Autodesk Inventor part; units mm, degrees
ref_plane "Płaszczyzna konstrukcyjna1" through (0, 0, 17) normal (-1, 0, 0) x (0, 0, 1)
ref_plane "YZ Plane" through (0, 0, 0) normal (1, 0, 0) x (0, 1, 0)
ref_plane "XZ Plane" through (0, 0, 0) normal (0, 1, 0) x (-1, 0, 0)
sketch "Szkic1" plane through (0, 0, 0) normal (0, 1, 0) x (-1, 0, 0)
  line L0 (0, 17) -> (0, -17) construction
  line L1 (0, 0) -> (-17, 0)
  line L2 (0, 17) -> (0, 19)
  line L3 (0, -17) -> (0, -19)
  line L4 (-16.5569, 0) -> (-18.5569, 0)
  line L5 (0, 19) -> (0, 29)
  line L6 (0, 29) -> (-2, 29)
  line L7 (-2, 29) -> (-2, 18.7083)
  line L8 (0, -19) -> (0, -29)
  line L9 (0, -29) -> (-2, -29)
  line L10 (-2, -29) -> (-2, -18.8469)
  line L11 (-18.5573, 2.8889) -> (-18.5573, -3.1111)
  arc A0 (-2, 18.7083) -> (-18.5573, 2.8889) centre (-2.7215, 2.8889) ccw
  arc A1 (-18.5573, -3.1111) -> (-2, -18.8469) centre (-2.8011, -3.1111) ccw
  arc A2 (0, 17) -> (0, -17) centre (0.449, 0) ccw
  dimension "d0" = 34
  dimension "d1" = 17
  dimension "d2" = 2
  dimension "d3" = 2
  dimension "d4" = 2
  dimension "d5" = 10
  dimension "d6" = 2
  dimension "d7" = 10
  dimension "d8" = 2
  dimension "d41" = 6
ref_plane "Płaszczyzna konstrukcyjna1" through (0, 0, 17) normal (-1, 0, 0) x (0, 0, 1)
extrude "Wyciągnięcie proste3" add sketch "Szkic1" along normal blind 10
sketch "Szkic4" plane through (0, 0, -29) normal (-1, 0, 0) x (0, 0, 1)
  line L0 (10.1531, 0) -> (10.1531, 10)
  line L1 (10.1531, 5) -> (0, 5) construction
  line L2 (0, 0) -> (0, 10)
  line L3 (10.1531, 10) -> (0, 10)
  line L4 (5.0765, 10) -> (5.0765, 0) construction
  line L5 (10.1531, 0) -> (0, 0)
  line L6 (47.7083, 0) -> (47.7083, 10)
  line L7 (47.7083, 5) -> (58, 5) construction
  line L8 (58, 0) -> (58, 10)
  line L9 (46, 10) -> (58, 10)
  line L10 (52.8541, 10) -> (52.8541, 0) construction
  circle A0 centre (52.8541, 5) radius 3
  circle A1 centre (5.0765, 5) radius 3
  point P0 (29, 0)
  dimension "d45" = 6
  dimension "d46" = 6
hole "Otwór4" at (0, 5, -23.9235) at (0, 5, 23.8541) direction (1, 0, 0) diameter 4.9784 depth 19.05 tip angle 118
sketch "Szkic5" plane through (18.5573, 0, 2.8889) normal (1, 0, 0) x (0, 0, -1)
  line L0 (0, 10) -> (6, 10)
  line L1 (3, 10) -> (3, 0)
  line L2 (0, 0) -> (6, 0)
  line L3 (0, 0) -> (0, 10)
  line L4 (0, 5) -> (6, 5)
  line L5 (6, 0) -> (6, 10)
  circle A0 centre (3, 5) radius 3
  point P0 (2.8889, 0)
  dimension "d54" = 6
hole "Otwór5" at (18.5573, 5, -0.1111) direction (-1, 0, 0) diameter 4.9784 depth 19.05 tip angle 118
properties part number "obejma_fi32_L44"
Design review of the part built by this model. Coordinates are the model's own, in mm. A direction names the side the tool comes from. Give positions to 0.01 mm unless a question says otherwise; leave off trailing zeros. Loops run counter-clockwise (first coordinate to the right, second up) from the corner with the lowest first, then second, coordinate; pieces in that order, holes last. Notation, with made-up numbers: (16, 77.5) -> (29, 77.5) arc R23 cw to (29, 96.5) -> close; hole circle Ø4 at (76, 16). An arc over 180 degrees is marked (long way). One line per item, written item: value.
Q1. We need section A-A on x = 8.25. Give the boundary of the cut face in (y, z).
Numbers:
outline: (0, -17.9) -> (10, -17.9) -> (10, -14.61) -> (0, -14.61) -> close; (0, 14.61) -> (10, 14.61) -> (10, 17.73) -> (0, 17.73) -> close
Q2. Draft analysis for pull direction Y (two halves, no side actions). For faces 1 (the flat face through (1, 5, -29)), 2 (the flat face through (17, 10, 0)), 3 (the flat face through (17, 0, 0)), 4 (the cylindrical face through (17.44, 7.43, 0.43)), state which applies: pulls with the +Y half, pulls with the -Y half, needs draft (parallel to the pull), parting line crosses it, or undercut.
Numbers:
face 1: needs draft
face 2: pulls with the +Y half
face 3: pulls with the -Y half
face 4: undercut
Q3. For pin 1 Ø2 at (y, z) = (5.5, -5.5) entering from -X; pin 2 Ø1 at (y, z) = (3, 0.5) entering from +X; pin 3 Ø4 at (x, y) = (11, 1.5) entering from +Z; pin 4 Ø5 at (y, z) = (4.5, -24.5) entering from +X, all flat-tipped, find the tip position at first contact; note any pin that passes through.
Numbers:
pin 1: stops at x = 15.27
pin 2: stops at x = 18.56
pin 3: stops at z = 17.43
pin 4: stops at x = 2
Q4. We need section C-C on y = 5. Give the boundary of the cut face in (x, z), and give its area (3 significant figures).
Numbers:
outline: (0, -29) -> (2, -29) -> (2, -26.41) -> (0, -26.41) -> close; (0, -21.43) -> (2, -21.43) -> (2, -18.85) arc R15.76 ccw to (18.56, -3.11) -> (18.56, -2.6) -> (16.36, -2.6) arc R17.01 cw to (0, -17) -> close; (0, 17) arc R17.01 cw to (16.39, 2.38) -> (18.56, 2.38) -> (18.56, 2.89) arc R15.84 ccw to (2, 18.71) -> (2, 21.36) -> (0, 21.36) -> close; (0, 26.34) -> (2, 26.34) -> (2, 29) -> (0, 29) -> close
area: 162 mm^2
Q5. We need section B-B on z = 0. Give the boundary of the cut face in (x, y).
Numbers:
outline: (16.56, 0) -> (18.56, 0) -> (18.56, 2.51) -> (16.56, 2.51) -> close; (16.56, 7.49) -> (18.56, 7.49) -> (18.56, 10) -> (16.56, 10) -> close
Q6. Machinability: for faces 5 (the flat face through (0, 5, 20)), 6 (the flat face through (2, 3, 26)), which of the approach directions +Z, -Z, +X, -X, +Y, -Y give a long, thin tool a straight path to every point of the face, cutting with its end or side? Answer none if there is none.
Numbers:
face 5: +Z, -Z, -X, +Y, -Y
face 6: +Z, +X, +Y, -Y
Q7. For L1, parallel to X at y = 1.5, z = -20.5; L2, parallel to Z at x = 9.5, y = 5.5; L3, parallel to Z at x = 10.25, y = 9.25, list the stretches that pass through material, from the lowest coordinate up.
Numbers:
L1: x = 0 to 2
L2: z = -17.37 to -13.79, 13.79 to 17.2
L3: z = -17 to -13.22, 13.22 to 16.82
